Solid Edge part; units mm, degrees
sketch "Sketch1" plane through (0, 0, 0) normal (0, 0, -1) x (-1, 0, 0)
  line L0 (-2.8868, 5) -> (-5.7735, 0)
  line L1 (-5.7735, 0) -> (-2.8868, -5)
  line L2 (-2.8868, -5) -> (2.8868, -5)
  line L3 (2.8868, -5) -> (5.7735, 0)
  line L4 (5.7735, 0) -> (2.8868, 5)
  line L5 (2.8868, 5) -> (-2.8868, 5)
extrude "Protrusion1" add sketch "Sketch1" along normal blind 3
sketch "Sketch2" plane through (0, 0, -3) normal (0, 0, -1) x (0.5, -0.866, 0)
  circle A0 centre (0, 0) radius 3
extrude "Kihúzás_2" add sketch "Sketch2" along normal blind 12
chamfer "Letörés_1" distance 0.8 angle 45 1 edges at (-1.5, 2.5981, -15)
cosmetic_thread "Thread1"
sketch "Sketch3" plane through (0, 0, 0) normal (-1, 0, 0) x (0, -1, 0)
  line L0 (3.7699, 1.1319) -> (5.7205, -1.1833)
  line L1 (5.7205, -1.1833) -> (13.1885, -1.1833)
  line L2 (13.1885, -1.1833) -> (13.1885, 2.2239)
  line L3 (13.1885, 2.2239) -> (3.7699, 1.1319)
revolve "RevolvedCutout1" cut sketch "Sketch3" angle 360 about axis through (0, 0, 0) along (0, 0, 1)
properties material "Acél"
Build history of the part. All positions in model axes, mm. A direction names the side the tool comes from. Coordinates: 2 decimals unless noted, no trailing zeros. Order: outer loops, then holes, each group sorted by start corner. A loop starts at its lowest first (then second) coordinate and runs counter-clockwise, first axis right, second up. Notation, with made-up numbers: (46.25, 37) - (87.25, 37) arc R25 cw to (87.25, 50) - close; hole circle Ø8 at (27.25, 54). An arc over 180 degrees is marked (long way). Put each result on its own line as item: value.
1. Saw through at B-B (z = -2.75). Write the cut outline in (x, y), and give its area (3 significant figures).
Answer sheet:
outline: (-5.77, 0) - (-2.89, -5) - (2.89, -5) - (5.77, 0) - (2.89, 5) - (-2.89, 5) - close
area: 86.6 mm^2
2. Tool access for faces 1 (the face through (4.31, 2.535, -1.645)), 2 (the face through (-2.5, 2.3, -3)): list every direction of +Z, -Z, +X, -X, +Y, -Y with a clear straight run to the whole face (end or side of a thin tool).
Answer sheet:
face 1: +Z, -Z, +X, +Y
face 2: -Z
3. Probe line 1 along Z through (x, y) = (-0.5, -3.5); line 2 along Z through (x, y) = (-3, -4); line 3 along Y through (x, z) = (0.5, -12.25). List the from-to ranges inside material, lowest first. Write a range as [from, to].
Answer sheet:
line 1: z = [-3, 0]
line 2: z = [-3, -0.33]
line 3: y = [-2.96, 2.96]
4. Drop flat-ended pins along their axis: P1, Ø1.5, axis at y = 4, z = -7.5, coming from the +X side; P2, Ø1, axis at x = -1.5, z = -10.5, coming from the +Y side; P3, Ø1, axis at y = -0.5, z = -5.5, coming from the -X side. Give the stop position or say it passes through.
Answer sheet:
P1: passes through
P2: stops at y = 2.83
P3: stops at x = -3
5. Saw through at C-C (z = -7.75). Write the cut outline in (x, y), and give its area (3 significant figures).
Answer sheet:
outline: circle Ø6 at (0, 0)
area: 28.3 mm^2
6. Saw through at A-A (x = 0). Write the cut outline in (y, z).
Answer sheet:
outline: (-5, -3) - (-3, -3) - (-3, -14.2) - (-2.2, -15) - (2.2, -15) - (3, -14.2) - (3, -3) - (5, -3) - (5, -0.33) - (4.72, 0) - (-4.72, 0) - (-5, -0.33) - close
